Autodesk Inventor part; units mm, degrees
ref_plane "YZ Plane" through (0, 0, 0) normal (1, 0, 0) x (0, 1, 0)
ref_plane "XZ Plane" through (0, 0, 0) normal (0, 1, 0) x (-1, 0, 0)
ref_plane "XY Plane" through (0, 0, 0) normal (0, 0, 1) x (1, 0, 0)
sketch "스케치1" plane through (0, 0, 0) normal (0, 1, 0) x (-1, 0, 0)
  circle A0 centre (0, 0) radius 5
  dimension "d0" = 10
extrude "돌출1" add sketch "스케치1" along normal blind 30
sketch "스케치2" plane through (0, 0, 0) normal (0, -1, 0) x (1, 0, 0)
  circle A0 centre (0, 0) radius 8
  dimension "d3" = 16
extrude "돌출2" add sketch "스케치2" along normal blind 10
sketch "스케치3" plane through (0, -10, 0) normal (0, -1, 0) x (1, 0, 0)
  circle A0 centre (0, 0) radius 5 construction
  line L0 (4.6188, 0) -> (2.3094, -4)
  line L1 (2.3094, -4) -> (-2.3094, -4)
  line L2 (-2.3094, -4) -> (-4.6188, 0)
  line L3 (-4.6188, 0) -> (-2.3094, 4)
  line L4 (-2.3094, 4) -> (2.3094, 4)
  line L5 (2.3094, 4) -> (4.6188, 0)
  dimension "d6" = 8
extrude "돌출3" cut sketch "스케치3" against normal blind 5.5
chamfer "모따기1" distance 2 angle 45 1 edges at (5, 30, 0)
thread "스레드1"
properties part number "나사 10파이 30mm"
Design review of the part built by this model. Coordinates are the model's own, in mm. A direction names the side the tool comes from. Give positions to 0.01 mm unless a question says otherwise; leave off trailing zeros. Loops run counter-clockwise (first coordinate to the right, second up) from the corner with the lowest first, then second, coordinate; pieces in that order, holes last. Notation, with made-up numbers: M 40.5,67 L 63.5,67 A11 ccw 63.5,82 Z; hole C 2,59 d2. An arc over 180 degrees is marked long. Return JSON: item names as keys, results as strings. Group by question number.
Item 1: We need section B-B (y = 24.5). Give the boundary of the cut face in (x, z), and give its area (3 significant figures).
Item 2: We need section D-D (y = -0.5). Give the boundary of the cut face in (x, z), and give its area (3 significant figures).
Item 3: Tool access review of faces 4 (the flat face through (-4, -10, -2)), 5 (the cylindrical face through (1.08, 13.8, 4.88)), 6 (the flat face through (0, -7, -4)): name each direction out of +Z, -Z, +X, -X, +Y, -Y from which nothing blocks a thin tool from reaching the whole face with its end or side.
Item 4: We need section C-C (z = 6). Give the boundary of the cut face in (x, y), and give its area (3 significant figures).
Item 5: For probe 1 along Y at (x, z) = (-6.5, -2); probe 2 along Z at (x, y) = (3.75, -8); probe 3 along Y at (x, z) = (-2, 2), list the stretches that pass through material, from the lowest coordinate up.
Item 6: Mouldability with a two-part tool opening along Z and no side actions: class faces 1 (the flat face through (-0.1, 0, -5.2)), 2 (the flat face through (-3.48, -7.29, 1.97)), 3 (the cylindrical face through (-1.73, -4.93, 7.81)) as released by +Z, released by -Z, zero draft, split by the parting line, or undercut.
Item 7: We need section A-A (x = 0). Give the boundary of the cut face in (y, z), and give its area (3 significant figures).
Item 8: Insertion check: pin 1 Ø5 at (x, y) = (2.5, 2) entering from +Z; pin 2 Ø4 at (x, z) = (1, 0.5) entering from -Y; pin 3 Ø8 at (y, z) = (6.5, -4.5) entering from +X. Each pin has a flat end and moves straight along its axis. Give the tip position at first contact, or say it passes through.
Output:
{
 "1": {"outline": "C 0,0 d10", "area": "78.5 mm^2"},
 "2": {"outline": "C 0,0 d16", "area": "201 mm^2"},
 "3": {"face 4": "+Z, -Z, +X, -X, -Y", "face 5": "+Y", "face 6": "-Y"},
 "4": {"outline": "M -5.29,-10 L 5.29,-10 L 5.29,0 L -5.29,0 Z", "area": "106 mm^2"},
 "5": {"probe 1": "y = -10 to 0", "probe 2": "z = -7.07 to -1.5, 1.5 to 7.07", "probe 3": "y = -4.5 to 30"},
 "6": {"face 1": "zero draft", "face 2": "undercut", "face 3": "split by the parting line"},
 "7": {"outline": "M -10,-8 L 0,-8 L 0,-5 L 28,-5 L 30,-3 L 30,3 L 28,5 L 0,5 L 0,8 L -10,8 L -10,4 L -4.5,4 L -4.5,-4 L -10,-4 Z", "area": "412 mm^2"},
 "8": {"pin 1": "stops at z = 7.94", "pin 2": "stops at y = -4.5", "pin 3": "stops at x = 4.97"}
}
